from build123d import *

# Parameters (mm, degrees)
EXTRUDE_2_DEPTH = 5


with BuildPart() as part:
    # Эскиз4 → Бобышка-Вытянуть2 (new body)
    with BuildSketch(Plane.XY):
        Polygon((162, -18.92), (152.5, 58), (58.64, 58), (0, 38.59), (-58.64, 58), (-152.5, 58), (-162, -18.92), (-148.658722082, -23.671565122), (-87.19, -31.21617284), (-88.237138959, -42.15617284), (-40.597138959, -57.662313559), (40.597138959, -57.662313559), (88.237138959, -42.15617284), (87.19, -31.21617284), (148.658722082, -23.671565122), align=None)
        with BuildLine():
            Line((10.908195141, 11.626317085), (21.848195141, 15.513282482))
            Line((21.848195141, 15.513282482), (18.617591482, 3.873282482))
            ThreePointArc((18.617591482, 3.873282482), (20.785443003, -1.336165522), (21.525, -6.93))
            ThreePointArc((21.525, -6.93), (-5.593834478, -27.715443003), (-18.617591482, 3.873282482))
            Line((-18.617591482, 3.873282482), (-21.848195141, 15.513282482))
            Line((-21.848195141, 15.513282482), (-10.908195141, 11.626317085))
            ThreePointArc((-10.908195141, 11.626317085), (0, 14.595), (10.908195141, 11.626317085))
        make_face(mode=Mode.SUBTRACT)
    extrude(amount=EXTRUDE_2_DEPTH)


solid = part.part
Here's how the part is built. I have some questions about the finished solid (model axes, mm). A direction names the side the tool comes from. Round coordinates to 2 decimals unless told otherwise and drop trailing zeros. Write each loop counter-clockwise with the first axis right and the second up, starting at its lowest first coordinate (ties: lowest second). Pieces come first, ordered by that corner, then holes.
1. If we mould it in two halves opening along X, with no side actions, what happens to faces 1 (the flat face through (-2, 27, 5)), 2 (the flat face through (-28.91, 48.16, 2.46)), 3 (the flat face through (157.316, 19.002, 2.465))? For each: released by +X, released by -X, zero draft, split by the parting line, or undercut.
2. I need wall thicknesses on L1, parallel to X at y = -31.5, z = 2.55; L2, parallel to X at y = -6.93, z = 3.3 (3 decimals); L3, parallel to Y at x = 103.5, z = 1.7. Which ranges of each line are inside material? Lowest first, please.
3. Will these pins go through, and if not, where does the flat tip stop? pin 1 Ø1 at (y, z) = (-32, 3) entering from +X; pin 2 Ø8 at (x, y) = (-32, -36) entering from -Z; pin 3 Ø1.5 at (y, z) = (-34.5, 3) entering from +X.
4. Suppose I cut it at C-C (y = -37). List the corners of the cut face in (x, z) for me.
5. Suppose I cut it at B-B (y = 49). List the corners of the cut face in (x, z) for me, and give its area (3 significant figures).
6. For faces 4 (the flat face through (29.73, 48.43, 2.46)), 5 (the flat face through (-157.184, 20.078, 2.465)), which set-ups out of +Z, -Z, +X, -X, +Y, -Y let a thin tool reach every point of the face, with its end or its side?
7. Suppose I cut it at D-D (x = 65.5). List the corners of the cut face in (y, z) for me.
8. Suppose I cut it at A-A (z = 2.1). List the corners of the cut face in (x, y) for me (3 decimals), and give its area (3 significant figures).
Answer sheet:
1. face 1: zero draft
1. face 2: undercut
1. face 3: released by +X
2. L1: x = -87.22 to 87.22
2. L2: x = -160.519 to -21.525, 21.525 to 160.519
2. L3: y = -29.21 to 58
3. pin 1: stops at x = 87.31
3. pin 2: stops at z = 0
3. pin 3: stops at x = 87.58
4. outline: (-87.74, 0) - (87.74, 0) - (87.74, 5) - (-87.74, 5) - close
5. outline: (-153.61, 0) - (-31.45, 0) - (-31.45, 5) - (-153.61, 5) - close; (31.45, 0) - (153.61, 0) - (153.61, 5) - (31.45, 5) - close
5. area: 1,220 mm2
6. face 4: +Z, -Z, +Y
6. face 5: +Z, -Z, -X, +Y
7. outline: (-49.56, 0) - (58, 0) - (58, 5) - (-49.56, 5) - close
8. outline: (-162, -18.92) - (-148.659, -23.672) - (-87.19, -31.216) - (-88.237, -42.156) - (-40.597, -57.662) - (40.597, -57.662) - (88.237, -42.156) - (87.19, -31.216) - (148.659, -23.672) - (162, -18.92) - (152.5, 58) - (58.64, 58) - (0, 38.59) - (-58.64, 58) - (-152.5, 58) - close; hole (-21.848, 15.513) - (-18.618, 3.873) arc R21.525 ccw (long way) to (18.618, 3.873) - (21.848, 15.513) - (10.908, 11.626) arc R21.525 ccw to (-10.908, 11.626) - close
8. area: 28,700 mm2
